Geometry: final body of the model. Coordinates: model frame, mm. A direction names the side the tool comes from. Coordinates: 2 decimals unless noted, no trailing zeros. Order: outer loops, then holes, each group sorted by start corner. A loop starts at its lowest first (then second) coordinate and runs counter-clockwise, first axis right, second up. Notation, with made-up numbers: M 49,86.25 L 90,86.25 A34 ccw 90,122.25 Z; hole C 46.25,82 d9. An arc over 180 degrees is marked long. Use CSV: the item, a comma, the result in double quotes. Start each with the question number.
1. Set-up query: faces 4 (the flat face through (0, -15, 0)), 5 (the flat face through (-33, -31, -9)), 6 (the flat face through (1.85, 5, 2)), 7 (the cylindrical face through (-64.086, -2.681, -6.466)), 8 (the flat face through (-29, -34, -6)). Return all of +Z, -Z, +X, -X, +Y, -Y with unobstructed straight access to the full face (end or side cutting, diameter ignored); none if empty.
2. Section query A-A on y = -11. Return the cut outline in (x, z).
3. Pull-direction query (X, two-part tool) for faces 1 (the cylindrical face through (-63, 9, 0)), 2 (the cylindrical face through (-35, -32, 0)), 3 (the flat face through (-61.85, 5, 2)); classes: pulls with the +X half, pulls with the -X half, needs draft (parallel to the pull), parting line crosses it, or undercut.
4. Section query D-D on y = 3. Return the cut outline in (x, z), and give its area (3 significant figures).
5. Section query C-C on x = -30. Return the cut outline in (y, z).
6. Section query B-B on z = 0. Return the cut outline in (x, y).
7. Material intervals for line 1 (Z direction, x = -30, y = -32); line 2 (Y direction, x = -63.3, z = 0); line 3 (X direction, y = -11, z = 2.5), sorted ascending.
8. First-contact query: P1, Ø7, axis at y = -1, z = 2, coming from the -X side; P2, Ø4, axis at x = -16, y = -29, coming from the -Z side. Flat tips, straight axial feed; report the tip coordinate or a pass-through.
from build123d import *

# Parameters (mm, degrees)
SKETCH1_R           = 9
SKETCH1_R_2         = 5
BOSS_EXTRUDE1_DEPTH = 6.26
BOSS_EXTRUDE2_DEPTH = 6.26
SKETCH2_R           = 7
CUT_EXTRUDE1_DEPTH  = 4.41
SKETCH4_W           = 36.26
SKETCH4_H           = 18
BOSS_EXTRUDE3_DEPTH = 4
SKETCH5_R           = 5
CUT_EXTRUDE2_DEPTH  = 5


with BuildPart() as part:
    # Sketch1 → Boss-Extrude1 (new body)
    with BuildSketch(Plane(origin=(0, 0, 0), x_dir=(0, 0, -1), z_dir=(1, 0, 0))):
        Circle(SKETCH1_R)
        Circle(SKETCH1_R_2, mode=Mode.SUBTRACT)
    extrude(amount=BOSS_EXTRUDE1_DEPTH)

    # Sketch3 → Boss-Extrude2 (add)
    with BuildSketch(Plane.ZY):
        with BuildLine():
            Line((-9, 0), (-9, -30))
            Line((-9, -30), (9, -30))
            Line((9, -30), (9, 0))
            Line((9, 0), (5, 0))
            ThreePointArc((5, 0), (0, -5), (-5, 0))
            Line((-5, 0), (-9, 0))
        make_face()
    extrude(amount=-BOSS_EXTRUDE2_DEPTH)

    # Sketch2 → Cut-Extrude1 (cut)
    with BuildSketch(Plane(origin=(6.26, 0, 0), x_dir=(0, 0, -1), z_dir=(1, 0, 0))):
        Circle(SKETCH2_R)
    extrude(amount=-CUT_EXTRUDE1_DEPTH, mode=Mode.SUBTRACT)

    # Sketch4 → Boss-Extrude3 (add)
    with BuildSketch(Plane.XZ.offset(30)):
        with Locations((-11.87, 0)):
            Rectangle(SKETCH4_W, SKETCH4_H)
    extrude(amount=BOSS_EXTRUDE3_DEPTH)

    # Mirror2: part across plane


with BuildPart() as part_1:
    add(part.part)
    add(part.part.mirror(Plane(origin=(-30, -34, 9), x_dir=(0, 0, 1), z_dir=(1, 0, 0))))

    # Sketch5 → Cut-Extrude2 (cut, through all)
    with BuildSketch(Plane(origin=(0, -30, 0), x_dir=(1, 0, 0), z_dir=(0, 1, 0))):
        with Locations((-30, 0)):
            Circle(SKETCH5_R)
    extrude(amount=-CUT_EXTRUDE2_DEPTH, mode=Mode.SUBTRACT)


solid = part_1.part
Results list:
1,face 4,"+Z, -Z, +Y"
1,face 5,"-Z, +X, -X, +Y, -Y"
1,face 6,"+X"
1,face 7,"-X"
1,face 8,"+Z, -Z, +X, -X, -Y"
2,outline,"M -66.26,-9 L -60,-9 L -60,9 L -66.26,9 Z; M 0,-9 L 6.26,-9 L 6.26,9 L 0,9 Z"
3,face 1,"needs draft"
3,face 2,"undercut"
3,face 3,"pulls with the -X half"
4,outline,"M -66.26,-8.49 L -60,-8.49 L -60,-4 L -61.85,-4 L -61.85,-6.32 L -66.26,-6.32 Z; M -66.26,6.32 L -61.85,6.32 L -61.85,4 L -60,4 L -60,8.49 L -66.26,8.49 Z; M 0,-8.49 L 6.26,-8.49 L 6.26,-6.32 L 1.85,-6.32 L 1.85,-4 L 0,-4 Z; M 0,4 L 1.85,4 L 1.85,6.32 L 6.26,6.32 L 6.26,8.49 L 0,8.49 Z"
4,area,"71.3 mm²"
5,outline,"M -34,-9 L -30,-9 L -30,-5 L -34,-5 Z; M -34,5 L -30,5 L -30,9 L -34,9 Z"
6,outline,"M -66.26,-34 L -35,-34 L -35,-30 L -60,-30 L -60,-5 L -61.85,-5 L -61.85,-7 L -66.26,-7 Z; M -66.26,7 L -61.85,7 L -61.85,5 L -60,5 L -60,9 L -66.26,9 Z; M -25,-34 L 6.26,-34 L 6.26,-7 L 1.85,-7 L 1.85,-5 L 0,-5 L 0,-30 L -25,-30 Z; M 0,5 L 1.85,5 L 1.85,7 L 6.26,7 L 6.26,9 L 0,9 Z"
7,line 1,"z = -9 to -5, 5 to 9"
7,line 2,"y = -34 to -7, 7 to 9"
7,line 3,"x = -66.26 to -60, 0 to 6.26"
8,P1,"stops at x = -61.85"
8,P2,"stops at z = -9"
